Input: part model. Units: mm. Frame: model coordinates. A direction names the side the tool comes from. Coordinates: 2 decimals unless noted, no trailing zeros. Write each loop counter-clockwise with the first axis right and the second up, starting at its lowest first coordinate (ties: lowest second). Pieces come first, ordered by that corner, then holes.
from build123d import *

# Parameters (mm, degrees)
SKETCH1_W           = 50.8
SKETCH1_H           = 25.4
SKETCH1_W_2         = 45.72
SKETCH1_H_2         = 20.32
BOSS_EXTRUDE1_DEPTH = 279.4
SKETCH2_R           = 6.35
SKETCH2_R_2         = 12.7
CUT_EXTRUDE1_DEPTH  = 286.114292872
SKETCH3_R           = 6.35
CUT_EXTRUDE2_DEPTH  = 286.114292872


with BuildPart() as part:
    # Sketch1 → Boss-Extrude1 (new body)
    with BuildSketch(Plane(origin=(0, 0, 0), x_dir=(1, 0, 0), z_dir=(0, 1, 0))):
        with Locations((25.4, 12.7)):
            Rectangle(SKETCH1_W, SKETCH1_H)
        with Locations((25.4, 12.7)):
            Rectangle(SKETCH1_W_2, SKETCH1_H_2, mode=Mode.SUBTRACT)
    extrude(amount=BOSS_EXTRUDE1_DEPTH)

    # Sketch2 → Cut-Extrude1 (cut, through all)
    with BuildSketch(Plane.XY):
        with Locations((12.7, 25.4)):
            Circle(SKETCH2_R)
        with Locations((25.4, 254)):
            Circle(SKETCH2_R_2)
    extrude(amount=-CUT_EXTRUDE1_DEPTH, mode=Mode.SUBTRACT)

    # Sketch3 → Cut-Extrude2 (cut, through all)
    with BuildSketch(Plane(origin=(0, 0, -25.4), x_dir=(-1, 0, 0), z_dir=(0, 0, -1))):
        with Locations((-38.1, 76.2)):
            Circle(SKETCH3_R)
    extrude(amount=-CUT_EXTRUDE2_DEPTH, mode=Mode.SUBTRACT)


solid = part.part
Item 1: Pull-direction query (X, two-part tool) for faces 1 (the face through (25, 138, 0)), 2 (the face through (50.8, 138, -13)), 3 (the face through (0, 138, -13)), 4 (the face through (25, 138, -22.86)); classes: released by +X, released by -X, zero draft, split by the parting line, or undercut.
Item 2: Access query for faces 5 (the face through (7.66, 21.54, -1.25)), 6 (the face through (48.26, 138, -13)). Directions: +Z, -Z, +X, -X, +Y, -Y. A direction counts if a zero-diameter tool reaches every point of the face in a straight line with its end or side. Return the directions, or none.
Item 3: Material intervals for line 1 (Z direction, x = 47, y = 129); line 2 (X direction, y = 133, z = -3.25); line 3 (Y direction, x = 25.4, z = -23.6), sorted ascending.
Item 4: Section query D-D, the plane y = 23. Return loops of the section in (x, z).
Item 5: Section query A-A, the plane z = -12. Return loops of the section in (x, y).
Item 6: Section query C-C, the plane y = 136. Return loops of the section in (x, z), then the cut area to 3 significant figures.
Item 7: Section query B-B, the plane x = 25.4. Return loops of the section in (y, z), then the cut area to 3 significant figures.
The answers:
1. face 1: zero draft
1. face 2: released by +X
1. face 3: released by -X
1. face 4: undercut
2. face 5: +Z, -Z
2. face 6: +Y, -Y
3. line 1: z = -25.4 to -22.86, -2.54 to 0
3. line 2: x = 0 to 2.54, 48.26 to 50.8
3. line 3: y = 0 to 241.3, 266.7 to 279.4
4. outline: (0, -25.4) - (6.82, -25.4) - (6.82, -22.86) - (2.54, -22.86) - (2.54, -2.54) - (6.82, -2.54) - (6.82, 0) - (0, 0) - close; (18.58, -25.4) - (50.8, -25.4) - (50.8, 0) - (18.58, 0) - (18.58, -2.54) - (48.26, -2.54) - (48.26, -22.86) - (18.58, -22.86) - close
5. outline: (0, 0) - (2.54, 0) - (2.54, 279.4) - (0, 279.4) - close; (48.26, 0) - (50.8, 0) - (50.8, 279.4) - (48.26, 279.4) - close
6. outline: (0, -25.4) - (50.8, -25.4) - (50.8, 0) - (0, 0) - close; hole (2.54, -22.86) - (48.26, -22.86) - (48.26, -2.54) - (2.54, -2.54) - close
6. area: 361 mm2
7. outline: (0, -25.4) - (241.3, -25.4) - (241.3, -22.86) - (0, -22.86) - close; (0, -2.54) - (241.3, -2.54) - (241.3, 0) - (0, 0) - close; (266.7, -25.4) - (279.4, -25.4) - (279.4, -22.86) - (266.7, -22.86) - close; (266.7, -2.54) - (279.4, -2.54) - (279.4, 0) - (266.7, 0) - close
7. area: 1,290 mm2
